from build123d import *

# Parameters (mm, degrees)
ESQUISSE1_R             = 7.5
BOSS_EXTRU_1_DEPTH      = 15
CHANFREIN1_SIZE         = 1
CONG_1_R                = 0.2
ESQUISSE2_R             = 8.1
ENL_V_MAT_EXTRU_1_DEPTH = 1
ENL_V_START             = -1
ESQUISSE3_R             = 8.1
ENL_V_MAT_EXTRU_2_DEPTH = 1
TROU_TARAUD_M41_D       = 3.3


with BuildPart() as part:
    # Esquisse1 → Boss.-Extru.1 (new, symmetric)
    with BuildSketch(Plane.XY):
        Polygon((5.6, 0.5), (-5.6, 0.5), (-6.1, 0), (-17.1, 0), (-17.1, 6), (-16.2, 6.9), (-16.2, 17.8), (-8, 17.8), (-4, 21.8), (4, 21.8), (8, 17.8), (16.2, 17.8), (16.2, 6.9), (17.1, 6), (17.1, 0), (6.1, 0), align=None)
        with Locations((0, 10.9)):
            Circle(ESQUISSE1_R, mode=Mode.SUBTRACT)
    extrude(amount=BOSS_EXTRU_1_DEPTH, both=True)

    # Chanfrein1
    chanfrein1_edges = [part.edges().sort_by_distance(p)[0] for p in [
        (-17.1, 0, 0),
        (-16.2, 17.8, 0),
        (16.2, 17.8, 0),
        (17.1, 0, 0),
    ]]
    chamfer(chanfrein1_edges, length=CHANFREIN1_SIZE)

    # Congé1
    cong_1_edges = [part.edges().sort_by_distance(p)[0] for p in [
        (6.1, 0, 0),
        (5.6, 0.5, 0),
        (-5.6, 0.5, 0),
        (-6.1, 0, 0),
        (-17.1, 6, 0),
        (-16.2, 6.9, 0),
        (-8, 17.8, 0),
        (-4, 21.8, 0),
        (4, 21.8, 0),
        (8, 17.8, 0),
        (16.2, 6.9, 0),
        (17.1, 6, 0),
        (17.1, 1, 0),
        (16.1, 0, 0),
        (-16.1, 0, 0),
        (-17.1, 1, 0),
        (-16.2, 16.8, 0),
        (-15.2, 17.8, 0),
        (15.2, 17.8, 0),
        (16.2, 16.8, 0),
    ]]
    fillet(cong_1_edges, radius=CONG_1_R)

    # Esquisse2 → Enlèv. mat.-Extru.1 (cut)
    with BuildSketch(Plane.XY.offset(13)):
        with Locations((0, 10.9)):
            Circle(ESQUISSE2_R)
    extrude(amount=-ENL_V_MAT_EXTRU_1_DEPTH, mode=Mode.SUBTRACT)

    # Esquisse3 → Enlèv. mat.-Extru.2 (cut)
    with BuildSketch(Plane(origin=(0, 0, -13), x_dir=(-1, 0, 0), z_dir=(0, 0, -1)).offset(ENL_V_START)):
        with Locations(Location((0, 10.9, 0), (0, 0, 180))):
            Circle(ESQUISSE3_R)
    extrude(amount=ENL_V_MAT_EXTRU_2_DEPTH, mode=Mode.SUBTRACT)

    # Trou taraudé M41 (through all)
    with Locations(Plane(origin=(0, 0, 0), x_dir=(-1, 0, 0), z_dir=(0, -1, 0))):
        with Locations((-12, -8), (12, -8), (12, 8), (-12, 8)):
            Hole(TROU_TARAUD_M41_D / 2)


solid = part.part
Source: CAD feature listing. Evaluate the final solid. Frame: model axes, mm. A direction names the side the tool comes from. Coordinates: 2 decimals unless noted, no trailing zeros. Order: outer loops, then holes, each group sorted by start corner. A loop starts at its lowest first (then second) coordinate and runs counter-clockwise, first axis right, second up. Notation, with made-up numbers: M -9.75,0.5 L 26.25,0.5 A3 cw 26.25,4.5 Z; hole C 72.25,50 d5. An arc over 180 degrees is marked long. Write each question's results on one line, items separated by ' | '. Start each with the question number.
1. Reachability of faces 1 (the face through (4, 4, 15)), 2 (the face through (16.2, 12, 0)), 3 (the face through (-16.2, 12, 0)), 4 (the face through (-1.756, 18.807, -12.493)), 5 (the face through (0, 0.5, 0)) from +Z, -Z, +X, -X, +Y, -Y: full face, straight path, thin tool, end or side. Return the list, or none.
2. Draft query along Y for faces 6 (the face through (5, 5, 13)), 7 (the face through (11, 0, 0)), 8 (the face through (12, 17.8, 0)). Return one class per face: +Y half, -Y half, draft (parallel to the pull), parting line (faces both ways), or undercut.
3. Section A-A, the plane y = 10.9. Return the cut outline in (x, z).
4. Section B-B, the plane x = 0. Return the cut outline in (y, z).
5. Material intervals for L1, parallel to Z at x = -12, y = 8.5; L2, parallel to Y at x = 0, z = 13.7; L3, parallel to X at y = 8.75, z = 8, sorted ascending.
6. Section C-C, the plane x = -12. Return the cut outline in (y, z).
7. Section D-D, the plane z = 8. State how many separate pieces and enclosed holes the cut face has, then the cut area to 3 significant figures.
8. Pin query (flat end, axial travel): pin 1 (4.5 mm diameter, centred on x = -12, z = -8, fed in from +Y); pin 2 (2 mm diameter, centred on x = 4.5, z = -5, fed in from -Y); pin 3 (3 mm diameter, centred on y = 13.5, z = 4.5, fed in from -X). Return the tip coordinate at first contact, or that it passes through.
Solution:
1) face 1: +Z, +X, -X, +Y, -Y | face 2: +Z, -Z, +X, +Y | face 3: +Z, -Z, -X, +Y | face 4: none | face 5: +Z, -Z, -Y
2) face 6: undercut | face 7: -Y half | face 8: +Y half
3) outline: M -16.2,-15 L -7.5,-15 L -7.5,-13 L -8.1,-13 L -8.1,-12 L -7.5,-12 L -7.5,12 L -8.1,12 L -8.1,13 L -7.5,13 L -7.5,15 L -16.2,15 Z; M 7.5,-15 L 16.2,-15 L 16.2,15 L 7.5,15 L 7.5,13 L 8.1,13 L 8.1,12 L 7.5,12 L 7.5,-12 L 8.1,-12 L 8.1,-13 L 7.5,-13 Z; hole C -12,-8 d3.3; hole C -12,8 d3.3; hole C 12,-8 d3.3; hole C 12,8 d3.3
4) outline: M 0.5,-15 L 3.4,-15 L 3.4,-13 L 2.8,-13 L 2.8,-12 L 3.4,-12 L 3.4,12 L 2.8,12 L 2.8,13 L 3.4,13 L 3.4,15 L 0.5,15 Z; M 18.4,-15 L 21.8,-15 L 21.8,15 L 18.4,15 L 18.4,13 L 19,13 L 19,12 L 18.4,12 L 18.4,-12 L 19,-12 L 19,-13 L 18.4,-13 Z
5) L1: -15 to -9.65, -6.35 to 6.35, 9.65 to 15 | L2: 0.5 to 3.4, 18.4 to 21.8 | L3: -16.2 to -13.65, -10.35 to -7.19, 7.19 to 10.35, 13.65 to 16.2
6) outline: M 0,-15 L 17.8,-15 L 17.8,-9.65 L 0,-9.65 Z; M 0,-6.35 L 17.8,-6.35 L 17.8,6.35 L 0,6.35 Z; M 0,9.65 L 17.8,9.65 L 17.8,15 L 0,15 Z
7) separate pieces: 3 | enclosed holes: 1 | area: 334 mm²
8) pin 1: y = 17.8 | pin 2: y = 0.5 | pin 3: x = -16.2
